Here's how the part is built. I have some questions about the finished solid (model axes, mm). A direction names the side the tool comes from. Coordinates: 2 decimals unless noted, no trailing zeros. Write each loop counter-clockwise with the first axis right and the second up, starting at its lowest first coordinate (ties: lowest second). Pieces come first, ordered by that corner, then holes.
Item 1: If we section it at B-B (y = 1.6): Please give me the cut outline in (x, z).
Item 2: If we section it at C-C (z = -8): Please give me the cut outline in (x, y), then the cut area to 3 significant figures.
Item 3: We'd pull the mould along Z, two halves only. Please class faces 4 (the face through (-9, 1, 32)), 5 (the face through (11.21, 1.479, 4.574)), 6 (the face through (0, 0, 9)): +Z half, -Z half, draft (parallel to the pull), parting line (faces both ways), or undercut.
Item 4: If we section it at D-D (x = 10.5): Please give me the cut outline in (y, z).
Item 5: For faces 1 (the face through (12.6, 1, 6)), 2 (the face through (9, 1, 32)), 3 (the face through (-7.88, 1.48, -6.18)), which set-ups out of +Z, -Z, +X, -X, +Y, -Y let a thin tool reach every point of the face, with its end or its side?
Item 6: If I drill on line 1 (X direction, y = 2.15, z = 3.8); line 2 (X direction, y = 2.05, z = 1); line 3 (X direction, y = 2.1, z = -8.5), over which ranges is the centre line in solid material (lowest first)?
Item 7: I'm going to push flat-ended pins straight in: pin 1 Ø1.5 at (x, z) = (-6.5, -6) entering from -Y; pin 2 Ø1.5 at (x, y) = (8.5, 2) entering from +Z. Where does each tip first touch, or does it pass through?
Item 8: If we section it at A-A (x = 6): Please give me the cut outline in (y, z), then the cut area to 3 significant figures.
from build123d import *

# Parameters (mm, degrees)
BOSS_EXTRUDE1_DEPTH = 3
SKETCH2_R           = 1.05
CUT_EXTRUDE1_DEPTH  = 10
CUT_EXTRUDE4_DEPTH  = 10
BOSS_EXTRUDE2_DEPTH = 3


with BuildPart() as part:
    # Sketch1 → Boss-Extrude1 (new body)
    with BuildSketch(Plane(origin=(0, 0, 0), x_dir=(1, 0, 0), z_dir=(0, 1, 0))):
        Polygon((-12.6, -12), (-12.6, -32), (-5, -32), (-5, -35), (0, -35), (5, -35), (5, -32), (12.6, -32), (12.6, -12), (12.6, 12), (-12.6, 12), align=None)
    extrude(amount=BOSS_EXTRUDE1_DEPTH)

    # Sketch2 → Cut-Extrude1 (cut)
    with BuildSketch(Plane.XZ):
        with Locations(Location((10.5, -8.5, 0), (0, 0, 270))):
            Circle(SKETCH2_R)
        with Locations(Location((-10.5, -8.5, 0), (0, 0, 270))):
            Circle(SKETCH2_R)
        with Locations(Location((-10.5, 3.8, 0), (0, 0, 270))):
            Circle(SKETCH2_R)
        with Locations(Location((10.5, 3.8, 0), (0, 0, 270))):
            Circle(SKETCH2_R)
    extrude(amount=-CUT_EXTRUDE1_DEPTH, mode=Mode.SUBTRACT)

    # Sketch5 → Cut-Extrude4 (cut)
    with BuildSketch(Plane(origin=(0, 0, 0), x_dir=(-1, 0, 0), z_dir=(0, -1, 0))):
        with BuildLine():
            Line((-10, 5.035898385), (-10, -1.863508327))
            Line((-10, -1.863508327), (-10, -2.070838353))
            Line((-10, -2.070838353), (-8.7, -3.8))
            Line((-8.7, -3.8), (-8.7, -5.6))
            Line((-8.7, -5.6), (8.7, -5.6))
            Line((8.7, -5.6), (8.7, -3.8))
            ThreePointArc((8.7, -3.8), (9.061250543, -2.718334617), (10, -2.070838353))
            Line((10, -2.070838353), (10, -1.863508327))
            Line((10, -1.863508327), (10, 5.035898385))
            ThreePointArc((10, 5.035898385), (7.854248689, 6.208712153), (7, 8.5))
            Line((7, 8.5), (7, 12))
            Line((7, 12), (-7, 12))
            Line((-7, 12), (-7, 8.5))
            ThreePointArc((-7, 8.5), (-7.854248689, 6.208712153), (-10, 5.035898385))
        make_face()
    extrude(amount=-CUT_EXTRUDE4_DEPTH, mode=Mode.SUBTRACT)

    # Sketch6 → Boss-Extrude2 (add)
    with BuildSketch(Plane.XZ):
        Polygon((7, -12), (7, -14), (-7, -14), (-7, -12), (-12.6, -12), (-12.6, -18.4), (12.6, -18.4), (12.6, -12), align=None)
    extrude(amount=-BOSS_EXTRUDE2_DEPTH)


solid = part.part
Answer list:
1. outline: (-12.6, -18.4) - (12.6, -18.4) - (12.6, 32) - (5, 32) - (5, 35) - (-5, 35) - (-5, 32) - (-12.6, 32) - close; hole circle Ø2.1 at (-10.5, -8.5); hole circle Ø2.1 at (-10.5, 3.8); hole (-10, -5.04) arc R3.5 cw to (-7, -8.5) - (-7, -14) - (7, -14) - (7, -8.5) arc R3.5 cw to (10, -5.04) - (10, 2.07) - (8.7, 3.8) - (8.7, 5.6) - (-8.7, 5.6) - (-8.7, 3.8) arc R1.8 cw to (-10, 2.07) - close; hole circle Ø2.1 at (10.5, -8.5); hole circle Ø2.1 at (10.5, 3.8)
2. outline: (-12.6, 0) - (-11.42, 0) - (-11.42, 3) - (-12.6, 3) - close; (-9.58, 0) - (-7.04, 0) - (-7.04, 3) - (-9.58, 3) - close; (7.04, 0) - (9.58, 0) - (9.58, 3) - (7.04, 3) - close; (11.42, 0) - (12.6, 0) - (12.6, 3) - (11.42, 3) - close
2. area: 22.3 mm2
3. face 4: +Z half
3. face 5: undercut
3. face 6: draft
4. outline: (0, -18.4) - (3, -18.4) - (3, -9.55) - (0, -9.55) - close; (0, -7.45) - (3, -7.45) - (3, 2.75) - (0, 2.75) - close; (0, 4.85) - (3, 4.85) - (3, 32) - (0, 32) - close
5. face 1: +Z, -Z, +X, +Y, -Y
5. face 2: +Z, +X, +Y, -Y
5. face 3: +Y, -Y
6. line 1: x = -12.6 to -11.55, -9.45 to -8.7, 8.7 to 9.45, 11.55 to 12.6
6. line 2: x = -12.6 to -10, 10 to 12.6
6. line 3: x = -12.6 to -11.55, -9.45 to -7, 7 to 9.45, 11.55 to 12.6
7. pin 1: passes through
7. pin 2: stops at z = 32
8. outline: (0, -18.4) - (3, -18.4) - (3, -14) - (0, -14) - close; (0, 5.6) - (3, 5.6) - (3, 32) - (0, 32) - close
8. area: 92.4 mm2
